from build123d import *

# Parameters (mm, degrees)
SKETCH1_W           = 40
SKETCH1_H           = 70
SKETCH1_R           = 7.5
BOSS_EXTRUDE1_DEPTH = 40
CUT_EXTRUDE1_DEPTH  = 20
SKETCH3_W           = 40
SKETCH3_H           = 50
CUT_EXTRUDE2_DEPTH  = 20
FILLET1_R           = 15


with BuildPart() as part:
    # Sketch1 → Boss-Extrude1 (new body)
    with BuildSketch(Plane.XY):
        with Locations((0, 15)):
            Rectangle(SKETCH1_W, SKETCH1_H)
        Circle(SKETCH1_R, mode=Mode.SUBTRACT)
    extrude(amount=BOSS_EXTRUDE1_DEPTH)

    # Sketch2 → Cut-Extrude1 (cut)
    with BuildSketch(Plane(origin=(0, 50, 0), x_dir=(1, 0, 0), z_dir=(0, 1, 0))):
        with BuildLine():
            ThreePointArc((7.5, -20), (2.870125743, -13.070903506), (-5.303300859, -14.696699141))
            Line((-5.303300859, -14.696699141), (5.303300859, -25.303300859))
            ThreePointArc((5.303300859, -25.303300859), (6.929096494, -22.870125743), (7.5, -20))
        make_face()
        with BuildLine():
            Line((5.303300859, -25.303300859), (-5.303300859, -14.696699141))
            ThreePointArc((-5.303300859, -14.696699141), (-5.303300859, -25.303300859), (5.303300859, -25.303300859))
        make_face()
    extrude(amount=-CUT_EXTRUDE1_DEPTH, mode=Mode.SUBTRACT)

    # Sketch3 → Cut-Extrude2 (cut)
    with BuildSketch(Plane.XY.offset(40)):
        with Locations((0, 5)):
            Rectangle(SKETCH3_W, SKETCH3_H)
    extrude(amount=-CUT_EXTRUDE2_DEPTH, mode=Mode.SUBTRACT)

    # Fillet1
    # the kernel refuses this fillet: 15 mm, written as the material it takes off along each edge
    with BuildSketch(Plane(origin=(20, -20, -37.5), x_dir=(0, 1, 0), z_dir=(0, 0, 1))) as fillet1_piece_1:
        with BuildLine():
            CenterArc((FILLET1_R, FILLET1_R), FILLET1_R, 180, 90)
            Line((0, FILLET1_R), (0, 0))
            Line((0, 0), (FILLET1_R, 0))
        make_face()
    extrude(amount=95, mode=Mode.SUBTRACT)
    with BuildSketch(Plane(origin=(-20, -20, -37.5), x_dir=(0, 1, 0), z_dir=(0, 0, 1))) as fillet1_piece_2:
        with BuildLine():
            CenterArc((FILLET1_R, -FILLET1_R), FILLET1_R, 90, 90)
            Line((0, -FILLET1_R), (0, 0))
            Line((0, 0), (FILLET1_R, 0))
        make_face()
    extrude(amount=95, mode=Mode.SUBTRACT)
    with BuildSketch(Plane(origin=(-20, 30, 77.5), x_dir=(0, 1, 0), z_dir=(0, 0, -1))) as fillet1_piece_3:
        with BuildLine():
            CenterArc((FILLET1_R, FILLET1_R), FILLET1_R, 180, 90)
            Line((0, FILLET1_R), (0, 0))
            Line((0, 0), (FILLET1_R, 0))
        make_face()
    extrude(amount=57.5, mode=Mode.SUBTRACT)
    with BuildSketch(Plane(origin=(20, 30, 77.5), x_dir=(0, 1, 0), z_dir=(0, 0, -1))) as fillet1_piece_4:
        with BuildLine():
            CenterArc((FILLET1_R, -FILLET1_R), FILLET1_R, 90, 90)
            Line((0, -FILLET1_R), (0, 0))
            Line((0, 0), (FILLET1_R, 0))
        make_face()
    extrude(amount=57.5, mode=Mode.SUBTRACT)


solid = part.part
The listing builds one solid part. Answer for the finished solid, in the listing's coordinates (mm). A direction names the side the tool comes from. Round coordinates to 2 decimals unless told otherwise and drop trailing zeros. Write each loop counter-clockwise with the first axis right and the second up, starting at its lowest first coordinate (ties: lowest second). Pieces come first, ordered by that corner, then holes. Notation, with made-up numbers: (66.5, 58) - (78.5, 58) arc R17 ccw to (78.5, 77) - close; hole circle Ø3 at (-17.75, 89). An arc over 180 degrees is marked (long way). Use one line per item in the form item = value. Start each with the question number.
Item 1: A cutting plane is placed at C-C (x = 0). Write down the section's boundary in (y, z).
Item 2: A cutting plane is placed at D-D (z = 37). Write down the section's boundary in (x, y).
Item 3: Determine the mould class of faces 6 (the flat face through (-20, 22, 11)), 7 (the cylindrical face through (-7.493, 0.33, 9.86)), 8 (the flat face through (0, 30, 33)) for opening direction X: +X half, -X half, draft (parallel to the pull), parting line (faces both ways), or undercut.
Item 4: Find the intervals of material crossed by line 1 (X direction, y = 0, z = 12); line 2 (Y direction, x = 0, z = 15); line 3 (Z direction, x = -12.5, y = 19), in increasing order. Write a range as [from, to].
Item 5: A cutting plane is placed at A-A (y = 0). Write down the section's boundary in (x, z).
Item 6: Flat-ended cylindrical pins translate along their axes: pin 1 Ø3 at (x, z) = (-4.5, 20) entering from +Y; pin 2 Ø12 at (x, y) = (0, 0) entering from -Z; pin 3 Ø3 at (x, z) = (-1, 34.5) entering from -Y; pin 4 Ø20 at (x, y) = (-6.5, 2.5) entering from +Z. Find the tip coordinate at first contact, or state that the pin passes through.
Item 7: A tool of negligible diameter and unlimited length cuts with its end or side. For faces 1 (the cylindrical face through (15.72, 34.51, 30.14)), 2 (the flat face through (0, 15, 0)), 3 (the cylindrical face through (-15.72, -15.49, 9.86)), 4 (the cylindrical face through (-15.49, 34.28, 30.14)), 5 (the flat face through (0, 30, 17)), from which of +Z, -Z, +X, -X, +Y, -Y can it reach the whole face along a straight path? Write none if from no direction.
Item 8: A cutting plane is placed at B-B (z = 23). Write down the section's boundary in (x, y), plus the area to 3 significant figures.
The answers:
q1.outline = (-20, 0) - (-7.5, 0) - (-7.5, 20) - (-20, 20) - close; (7.5, 0) - (50, 0) - (50, 12.5) - (30, 12.5) - (30, 20) - (7.5, 20) - close; (30, 27.5) - (50, 27.5) - (50, 40) - (30, 40) - close
q2.outline = (-20, 45) arc R15 ccw to (-5, 30) - (5, 30) arc R15 ccw to (20, 45) - (20, 50) - (-20, 50) - close
q3.face_6 = -X half
q3.face_7 = undercut
q3.face_8 = draft
q4.line_1 = [-20, -7.5], [7.5, 20]
q4.line_2 = [-20, -7.5], [7.5, 30]
q4.line_3 = [0, 20]
q5.outline = (-20, 0) - (-7.5, 0) - (-7.5, 20) - (-20, 20) - close; (7.5, 0) - (20, 0) - (20, 20) - (7.5, 20) - close
q6.pin_1 = 30
q6.pin_2 = through
q6.pin_3 = 30
q6.pin_4 = 20
q7.face_1 = +Z, +X, -Y
q7.face_2 = -Z, +X, -X, +Y, -Y
q7.face_3 = +Z, -Z, -X, -Y
q7.face_4 = +Z, -X, -Y
q7.face_5 = +Y
q8.outline = (-20, 45) arc R15 ccw to (-6.87, 30.12) - (-6.87, 50) - (-20, 50) - close; (6.87, 30.12) arc R15 ccw to (20, 45) - (20, 50) - (6.87, 50) - close
q8.area = 429 mm^2
